Verification items for this drawing (mm, ordinates from the low corner). Round coordinates to 2 decimals unless told otherwise and drop trailing zeros. Order: outer loops, then holes, each group sorted by start corner. A loop starts at its lowest first (then second) coordinate and runs counter-clockwise, first axis right, second up. Notation, with made-up numbers: (79, -18.5) - (85, -18.5) arc R16 cw to (85, 12.5) - close; hole circle Ø11 at (15.25, -20). An arc over 180 degrees is marked (long way). Use a Markdown table: item, result. Add a question column.
(1) Section check B-B on z = 1.1. Record the boundary of the cut face in (x, y) (1 decimal).
(2) Section check C-C on y = 200.5. Record the boundary of the cut face in (x, z) (1 decimal).
(3) Gauge pin test, flat ends, axial feed: P1, Ø5, axis at x = 122.5, y = 141.5, coming from the -Z side; P2, Ø2.5, axis at y = 217, z = 1.5, coming from the +X side; P3, Ø2.5, axis at y = 212.5, z = 2.5, coming from the +X side; P4, Ø2.5, axis at y = 218.5, z = 3.5, coming from the -X side. Record the tip position at first contact, or that the pin passes through.
(4) Thickness scan on line 1 along Y through (x, z) = (29, 1.8); line 2 along Y through (x, z) = (60, 0.35) (1 decimal); line 3 along Y through (x, z) = (39.5, 0.7) (1 decimal). Record the ranges inside material, lowest first. Write a range as [from, to].
(5) Section check D-D on x = 13. Record the boundary of the cut face in (y, z).
(6) Section check A-A on x = 64.5. Record the boundary of the cut face in (y, z) (1 decimal), then the cut area to 3 significant figures.
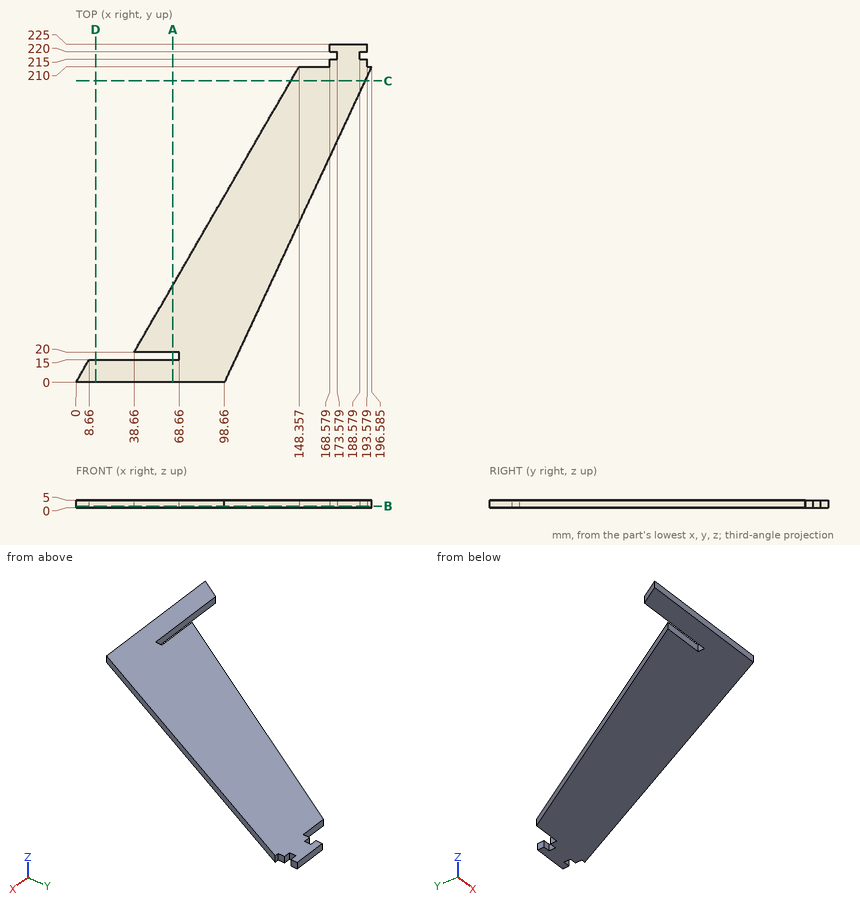
Check sheet entries:
| question | item | result |
|---|---|---|
| 1 | outline | (0, 0) - (98.7, 0) - (196.6, 210) - (193.6, 210) - (193.6, 215) - (188.6, 215) - (188.6, 220) - (193.6, 220) - (193.6, 225) - (168.6, 225) - (168.6, 220) - (173.6, 220) - (173.6, 215) - (168.6, 215) - (168.6, 210) - (148.4, 210) - (38.7, 20) - (68.7, 20) - (68.7, 15) - (8.7, 15) - close |
| 2 | outline | (142.9, 0) - (192.2, 0) - (192.2, 5) - (142.9, 5) - close |
| 3 | P1 | stops at z = 0 |
| 3 | P2 | stops at x = 188.58 |
| 3 | P3 | stops at x = 193.58 |
| 3 | P4 | stops at x = 173.58 |
| 4 | line 1 | y = [0, 15] |
| 4 | line 2 | y = [0, 15], [20, 57] |
| 4 | line 3 | y = [0, 15], [20, 21.5] |
| 5 | outline | (0, 0) - (15, 0) - (15, 5) - (0, 5) - close |
| 6 | outline | (0, 0) - (15, 0) - (15, 5) - (0, 5) - close; (20, 0) - (64.8, 0) - (64.8, 5) - (20, 5) - close |
| 6 | area | 299 mm2 |
